Work out the finished part from the listing and answer in its coordinate system (mm). Face numbers are marked on the shaded views. A direction names the side the tool comes from. Round coordinates to 2 decimals unless told otherwise and drop trailing zeros. Write each loop counter-clockwise with the first axis right and the second up, starting at its lowest first coordinate (ties: lowest second). Pieces come first, ordered by that corner, then holes.
1. Find section C-C (x = 0.75). Write down the section's boundary in (y, z).
2. Flat-ended cylindrical pins translate along their axes: pin 1 Ø0.8 at (x, y) = (-0.5, 2.5) entering from +Z; pin 2 Ø1.7 at (y, z) = (3, 8) entering from -X; pin 3 Ø1.6 at (x, y) = (5.5, 3) entering from +Z. Find the tip coordinate at first contact, or state that the pin passes through.
3. Find section B-B (y = 3). Write down the section's boundary in (x, z).
4. A tool of negligible diameter and unlimited length cuts with its end or side. For the marked faces 1, 2, 3, 4 and 5, from which of +Z, -Z, +X, -X, +Y, -Y can it reach the whole face along a straight path? Write none if from no direction.
5. Find section A-A (x = 2). Write down the section's boundary in (y, z), and give its area (3 significant figures).
6. Determine the mould class of the marked faces 6, 7 and 8 for opening direction Y: pulls with the +Y half, pulls with the -Y half, needs draft (parallel to the pull), parting line crosses it, or undercut.
7. Straight lines are drawn through the part: probe 1 along Y at (x, z) = (0, 8); probe 2 along Z at (x, y) = (-2.8, 3); probe 3 along Z at (x, y) = (-3.25, 2.5). For each, find the intervals that lie inside material, in ascending order.
8. Find section D-D (y = 5.75). Count the separate pieces of the cut face and the enclosed holes in it, and give its area (3 significant figures).
```python
from build123d import *

# Parameters (mm, degrees)
SKETCH1_W                   = 12
SKETCH1_H                   = 6
BOSS_EXTRUDE1_DEPTH         = 6
F_75_0_021_DIAMETER_HOLE1_D = 0.5334
SKETCH15_W                  = 6
SKETCH15_H                  = 6
BOSS_EXTRUDE2_DEPTH         = 7
FILLET4_R                   = 0.5
FILLET3_R                   = 1.5
SKETCH19_R                  = 1.35
CUT_EXTRUDE1_DEPTH          = 5.5
SKETCH16_R                  = 1.35
CUT_EXTRUDE2_DEPTH          = 5


with BuildPart() as part:
    # Sketch1 → Boss-Extrude1 (new body)
    with BuildSketch(Plane(origin=(0, 0, 0), x_dir=(1, 0, 0), z_dir=(0, 1, 0))):
        Rectangle(SKETCH1_W, SKETCH1_H)
    extrude(amount=BOSS_EXTRUDE1_DEPTH)

    # 75 _0.021_ Diameter Hole1 (through all)
    with Locations(Plane(origin=(0, 6, 0), x_dir=(1, 0, 0), z_dir=(0, 1, 0))):
        with Locations((0.7667, 0), (-0.7667, 0)):
            Hole(F_75_0_021_DIAMETER_HOLE1_D / 2)

    # Sketch15 → Boss-Extrude2 (add)
    with BuildSketch(Plane.XY.offset(3)):
        with Locations((0, 3)):
            Rectangle(SKETCH15_W, SKETCH15_H)
    extrude(amount=BOSS_EXTRUDE2_DEPTH)

    # Fillet4
    fillet4_edges = [part.edges().sort_by_distance(p)[0] for p in [
        (-4.5, 6, 3),
        (4.5, 0, 3),
        (4.5, 6, 3),
        (-4.5, 0, 3),
        (0, 0, -3),
        (0, 6, -3),
    ]]
    fillet(fillet4_edges, radius=FILLET4_R)

    # Fillet3
    # the kernel refuses this fillet: 1.5 mm, written as the material it adds along each edge
    with BuildSketch(Plane(origin=(3, 0.5, 3), x_dir=(1, 0, 0), z_dir=(0, 1, 0)), Plane(origin=(-3, 5.5, 3), x_dir=(-1, 0, 0), z_dir=(0, -1, 0))) as fillet3_piece_1:
        with BuildLine():
            CenterArc((FILLET3_R, -FILLET3_R), FILLET3_R, 90, 90)
            Line((0, -FILLET3_R), (0, 0))
            Line((0, 0), (FILLET3_R, 0))
        make_face()
    extrude(amount=5)
    with BuildSketch(Plane(origin=(3, 0.5, 2.5), x_dir=(0, 0.006283143965558622, 0.9999802608561372), z_dir=(0, -0.9999802608561372, 0.006283143965558622))) as fillet3_piece_2_section:
        with BuildLine():
            CenterArc((-0.5 - FILLET3_R, -FILLET3_R), FILLET3_R, 0, 90)
            Line((-0.5 - FILLET3_R, 0), (-0.5, 0))
            Line((-0.5, 0), (-0.5, -FILLET3_R))
        make_face()
    fillet3_piece_2 = revolve(axis=Axis((3, 0.5, 2.5), (-1, 0, 0)), revolution_arc=359.64, mode=Mode.PRIVATE)
    fillet3_piece_2 = split(fillet3_piece_2, bisect_by=Plane(origin=(3.567816549, 0, 2.882028447), z_dir=(0, 1, 0)), keep=Keep.TOP, mode=Mode.PRIVATE)
    add(fillet3_piece_2)
    with BuildSketch(Plane(origin=(3, 5.5, 2.5), x_dir=(0, -0.0062831439655592885, 0.9999802608561372), z_dir=(0, 0.9999802608561372, 0.0062831439655592885))) as fillet3_piece_3_section:
        with BuildLine():
            CenterArc((-0.5 - FILLET3_R, FILLET3_R), FILLET3_R, 270, 90)
            Line((-0.5 - FILLET3_R, 0), (-0.5, 0))
            Line((-0.5, 0), (-0.5, FILLET3_R))
        make_face()
    fillet3_piece_3 = revolve(axis=Axis((3, 5.5, 2.5), (1, 0, 0)), revolution_arc=359.64, mode=Mode.PRIVATE)
    fillet3_piece_3 = split(fillet3_piece_3, bisect_by=Plane(origin=(3.567816573, 6, 2.8820284), z_dir=(0, -1, 0)), keep=Keep.TOP, mode=Mode.PRIVATE)
    add(fillet3_piece_3)
    with BuildSketch(Plane(origin=(-3, 0.5, 2.5), x_dir=(0, 0, 1), z_dir=(0, 1, 0))) as fillet3_piece_4_section:
        with BuildLine():
            CenterArc((0.5 + FILLET3_R, -FILLET3_R), FILLET3_R, 90, 90)
            Line((0.5 + FILLET3_R, 0), (0.5, 0))
            Line((0.5, 0), (0.5, -FILLET3_R))
        make_face()
    fillet3_piece_4 = revolve(axis=Axis((-3, 0.5, 2.5), (1, 0, 0)), revolution_arc=359.64, mode=Mode.PRIVATE)
    fillet3_piece_4 = split(fillet3_piece_4, bisect_by=Plane(origin=(-3.567816642, 0, 2.882028407), z_dir=(0, 1, 0)), keep=Keep.TOP, mode=Mode.PRIVATE)
    add(fillet3_piece_4)
    with BuildSketch(Plane(origin=(-3, 5.5, 2.5), x_dir=(0, 0, 1), z_dir=(0, -1, 0))) as fillet3_piece_5_section:
        with BuildLine():
            CenterArc((0.5 + FILLET3_R, FILLET3_R), FILLET3_R, 180, 90)
            Line((0.5 + FILLET3_R, 0), (0.5, 0))
            Line((0.5, 0), (0.5, FILLET3_R))
        make_face()
    fillet3_piece_5 = revolve(axis=Axis((-3, 5.5, 2.5), (-1, 0, 0)), revolution_arc=359.64, mode=Mode.PRIVATE)
    fillet3_piece_5 = split(fillet3_piece_5, bisect_by=Plane(origin=(-3.567816642, 6, 2.882028407), z_dir=(0, -1, 0)), keep=Keep.TOP, mode=Mode.PRIVATE)
    add(fillet3_piece_5)

    # Sketch19 → Cut-Extrude1 (cut)
    with BuildSketch(Plane.ZY.offset(6)):
        with Locations((0, 3)):
            Circle(SKETCH19_R)
    cut_extrude1 = extrude(amount=-CUT_EXTRUDE1_DEPTH, mode=Mode.SUBTRACT)

    # Sketch16 → Cut-Extrude2 (cut)
    with BuildSketch(Plane.XY.offset(10)):
        with Locations((0, 3)):
            Circle(SKETCH16_R)
    extrude(amount=-CUT_EXTRUDE2_DEPTH, mode=Mode.SUBTRACT)

    # Mirror2: Cut-Extrude1 across plane
    add(cut_extrude1.mirror(Plane(origin=(0, 0, 0), x_dir=(0, 0, 1), z_dir=(1, 0, 0))), mode=Mode.SUBTRACT)


solid = part.part
```
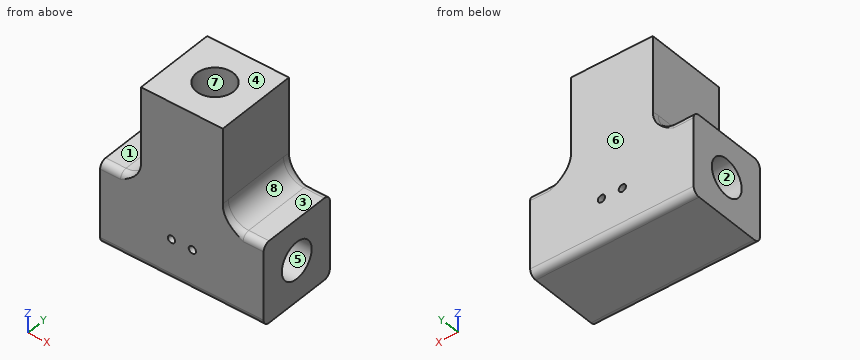
Worked answers:
1. outline: (0, -2.5) arc R0.5 ccw to (0.5, -3) - (5.5, -3) arc R0.5 ccw to (6, -2.5) - (6, -0.27) - (4.32, -0.27) arc R1.35 cw to (1.68, -0.27) - (0, -0.27) - close; (0, 0.27) - (1.68, 0.27) arc R1.35 cw to (4.32, 0.27) - (6, 0.27) - (6, 10) - (4.12, 10) - (4.12, 5) - (1.88, 5) - (1.88, 10) - (0, 10) - close
2. pin 1: stops at z = 5
2. pin 2: stops at x = -3
2. pin 3: stops at z = 3
3. outline: (-6, -3) - (6, -3) - (6, -1.35) - (0.5, -1.35) - (0.5, 1.35) - (6, 1.35) - (6, 3) - (4.5, 3) arc R1.5 cw to (3, 4.5) - (3, 10) - (1.35, 10) - (1.35, 5) - (-1.35, 5) - (-1.35, 10) - (-3, 10) - (-3, 4.5) arc R1.5 cw to (-4.5, 3) - (-6, 3) - (-6, 1.35) - (-0.5, 1.35) - (-0.5, -1.35) - (-6, -1.35) - close
4. face 1: +Z, -X, +Y, -Y
4. face 2: -X
4. face 3: +Z, +X, +Y, -Y
4. face 4: +Z, +X, -X, +Y, -Y
4. face 5: +X
5. outline: (0, -2.5) arc R0.5 ccw to (0.5, -3) - (5.5, -3) arc R0.5 ccw to (6, -2.5) - (6, 10) - (0, 10) - close; hole circle Ø2.7 at (3, 0)
5. area: 72.2 mm2
6. face 6: pulls with the +Y half
6. face 7: undercut
6. face 8: needs draft
7. probe 1: y = 0 to 1.65, 4.35 to 6
7. probe 2: z = -3 to -1.35, 1.35 to 10
7. probe 3: z = -3 to -1.25, 1.25 to 3.67
8. separate pieces: 1
8. enclosed holes: 2
8. area: 113 mm2
